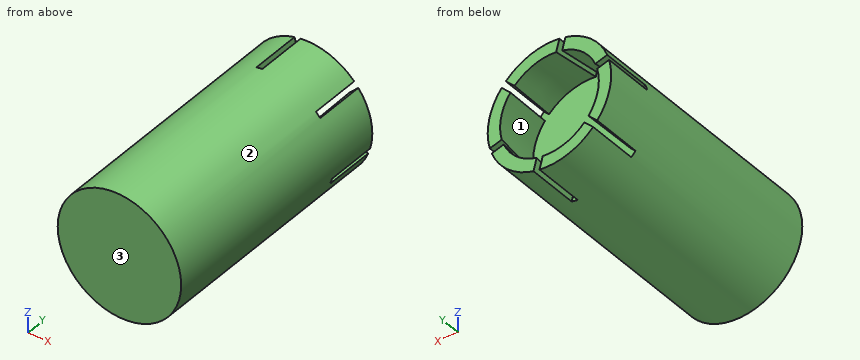
from build123d import *

# Parameters (mm, degrees)
SKETCH2_W             = 5
SKETCH2_H             = 20
SLOTS_START           = -4
SLOTS_DEPTH           = 4.5
SLOT_CIRPATTERN_COUNT = 6
SKETCH4_R             = 4
JOYSTICKHOLE_DEPTH    = 4
JOYSTICKHOLE_TAPER    = -6


with BuildPart() as part:
    # Sketch2 → Mount (revolve)
    with BuildSketch(Plane.XY):
        with Locations((2.5, -10)):
            Rectangle(SKETCH2_W, SKETCH2_H)
    revolve(axis=Axis((0, 5.533812346, 0), (0, -1, 0)))

    # Sketch3 → Slots (cut)
    with BuildSketch(Plane(origin=(0, 0, 0), x_dir=(1, 0, 0), z_dir=(0, 1, 0)).offset(SLOTS_START)):
        Polygon((-4.242640687, 4.242640687), (0, 0), (-0.353553391, -0.353553391), (-4.596194078, 3.889087297), align=None)
    slots = extrude(amount=SLOTS_DEPTH, mode=Mode.SUBTRACT)

    # Slot CirPattern: Slots ×6 about axis
    slot_cirpattern_axis = Axis((0, 0, 0), (0, 1, 0))
    for i in range(1, SLOT_CIRPATTERN_COUNT):
        add(slots.rotate(slot_cirpattern_axis, i * 360 / SLOT_CIRPATTERN_COUNT), mode=Mode.SUBTRACT)

    # Sketch4 → JoystickHole (cut)
    with BuildSketch(Plane(origin=(0, 0, 0), x_dir=(1, 0, 0), z_dir=(0, 1, 0))):
        Circle(SKETCH4_R)
    extrude(amount=-JOYSTICKHOLE_DEPTH, taper=JOYSTICKHOLE_TAPER, mode=Mode.SUBTRACT)


solid = part.part
Part model, mm, in its own coordinate system. Face numbers are marked on the shaded views. Coordinates: 2 decimals unless noted, no trailing zeros. Loops run counter-clockwise (first coordinate to the right, second up) from the corner with the lowest first, then second, coordinate; pieces in that order, holes last. Notation, with made-up numbers: (31.5, 47.25) -> (75.5, 47.25) arc R16 cw to (75.5, 75.25) -> close; hole circle Ø3 at (8.25, 64). An arc over 180 degrees is marked (long way). Use a Markdown table: item, result. Add a question column.
Item 1: Band-saw the part on B-B on x = 0. Write the cut outline in (y, z).
Item 2: Pull direction X, two halves, no side cores. Call the marked faces 1, 2 and 3: +X half, -X half, draft (parallel to the pull), parting line (faces both ways), or undercut.
Item 3: Band-saw the part on A-A on z = 0. Write the cut outline in (x, y), plus the area to 3 significant figures.
Item 4: Band-saw the part on C-C on y = -8.25. Write the cut outline in (x, z).
Item 5: Flat gauge pins, fed straight in: P1, Ø1.5, axis at y = -2.5, z = 3.5, coming from the +X side; P2, Ø1, axis at y = -14, z = -1, coming from the +X side; P3, Ø1, axis at x = 0, z = 2.5, coming from the +Y side. Where does each tip first touch, or does it go through?
Item 6: Probe probe 1 along Y at (x, z) = (-3.5, 1.75); probe 2 along Z at (x, y) = (-1.25, -8); probe 3 along X at (y, z) = (-2.5, -2). List the from-to ranges inside material, lowest first.
Geometry says:
| question | item | result |
|---|---|---|
| 1 | outline | (-20, -5) -> (0, -5) -> (0, -4) -> (-4, -4.42) -> (-4, 4.42) -> (0, 4) -> (0, 5) -> (-20, 5) -> close |
| 2 | face 1 | undercut |
| 2 | face 2 | parting line |
| 2 | face 3 | draft |
| 3 | outline | (-5, -20) -> (5, -20) -> (5, 0) -> (4, 0) -> (4.42, -4) -> (-4.42, -4) -> (-4, 0) -> (-5, 0) -> close |
| 3 | area | 166 mm² |
| 4 | outline | circle Ø10 at (0, 0) |
| 5 | P1 | x = 4.18 |
| 5 | P2 | x = 4.97 |
| 5 | P3 | y = -4 |
| 6 | probe 1 | -20 to -4 |
| 6 | probe 2 | -4.84 to 4.84 |
| 6 | probe 3 | -4.58 to -3.76, 3.76 to 4.58 |
